Could you check a few things on this model? Use its own coordinates, in mm. A direction names the side the tool comes from. Coordinates: 2 decimals unless noted, no trailing zeros. Loops run counter-clockwise (first coordinate to the right, second up) from the corner with the lowest first, then second, coordinate; pieces in that order, holes last. Notation, with made-up numbers: (-24, 85.5) - (-14, 85.5) arc R26 ccw to (-14, 122.5) - close; hole circle Ø4 at (76, 75.25). An arc over 180 degrees is marked (long way). One line per question, with ' | ' between items. Start each with the question number.
1. We'd pull the mould along X, two halves only. Please class faces 3 (the flat face through (3.59, 0.746, 5.54)), 4 (the flat face through (0, -5, 0)): pulls with the +X half, pulls with the -X half, needs draft (parallel to the pull), parting line crosses it, or undercut.
2. I want a section at A-A, the plane x = 0. Write out the boundary of the cut face in (y, z).
3. I want a section at D-D, the plane x = -5.5. Write out the boundary of the cut face in (y, z).
4. I'm going to push flat-ended pins straight in: P1, Ø1.1, axis at x = -3, y = 4, coming from the +Z side; P2, Ø1.2, axis at y = 3, z = 6, coming from the +X side; P3, Ø3, axis at x = -4, z = 3, coming from the +Y side; P4, Ø1, axis at y = -1.5, z = 2, coming from the +X side. Where does each tip first touch, or does it pass through?
5. I want a section at B-B, the plane y = 0. Write out the boundary of the cut face in (x, z).
6. Please list where these lines run through material, in increasing order: L1, parallel to Y at x = 0, z = 0.7; L2, parallel to Y at x = 0, z = 2; L3, parallel to X at y = -0.5, z = 5.75. Write a range as [from, to].
7. I want a section at C-C, the plane y = -2.75. Write out the boundary of the cut face in (x, z).
8. Which directions (+Z, -Z, +X, -X, +Y, -Y) give clear straight access to the entire face, cutting with the end or side of a thin tool? Please do faces 1 (the flat face through (3.6, 0.223, 5.54)), 2 (the cylindrical face through (3.65, -2.8, 0.74)).
from build123d import *

# Parameters (mm, degrees)
SKETCH1_R           = 5.6
SKETCH1_R_2         = 1.5
BOSS_EXTRUDE1_DEPTH = 6.3
SKETCH2_R           = 1.7
CUT_EXTRUDE1_DEPTH  = 0.7
SKETCH3_R           = 5.1
SKETCH3_R_2         = 2.2
CUT_EXTRUDE2_DEPTH  = 1.5
BOSS_EXTRUDE2_DEPTH = 1.5
SKETCH5_R           = 4.6
SKETCH5_R_2         = 2.5
CUT_EXTRUDE3_DEPTH  = 1.5
BOSS_EXTRUDE4_START = -6.3
SKETCH6_R           = 7.35
SKETCH6_R_2         = 5.6
BOSS_EXTRUDE4_DEPTH = 6.3


with BuildPart() as part:
    # Sketch1 → Boss-Extrude1 (new body)
    with BuildSketch(Plane.XY):
        Circle(SKETCH1_R)
        Circle(SKETCH1_R_2, mode=Mode.SUBTRACT)
    extrude(amount=BOSS_EXTRUDE1_DEPTH)

    # Sketch2 → Cut-Extrude1 (cut)
    with BuildSketch(Plane.XY.offset(6.3)):
        Circle(SKETCH2_R)
    extrude(amount=-CUT_EXTRUDE1_DEPTH, mode=Mode.SUBTRACT)

    # Sketch3 → Cut-Extrude2 (cut)
    with BuildSketch(Plane.XY.offset(6.3)):
        Circle(SKETCH3_R)
        Circle(SKETCH3_R_2, mode=Mode.SUBTRACT)
    extrude(amount=-CUT_EXTRUDE2_DEPTH, mode=Mode.SUBTRACT)

    # Sketch4 → Boss-Extrude2 (add)
    with BuildSketch(Plane.XY.offset(4.8)):
        Polygon((-0.9, 2.00748599), (-0.9, 5.019960159), (-0.9, 5.084289528), (-0.4, 5.084289528), (-0.4, 2.163330765), (-0.4, 2.00748599), align=None)
        Polygon((0.4, 5.084289528), (0.4, 2.163330765), (0.4, 2.00748599), (0.9, 2.00748599), (0.9, 5.019960159), (0.9, 5.084289528), align=None)
        Polygon((1.631117337, 1.476298152), (4.496150526, 2.407203865), (4.557331391, 2.427082733), (4.711839888, 1.951554475), (1.933843023, 1.048928577), (1.785625834, 1.000769893), align=None)
        Polygon((2.03283943, 0.23992468), (2.187347927, -0.235603578), (5.052381116, 0.695302136), (5.113561981, 0.715181004), (4.959053484, 1.190709262), (2.181056619, 0.288083364), align=None)
        Polygon((1.908085954, -1.095083555), (3.678773844, -3.532226353), (3.716585698, -3.584269905), (3.3120772, -3.878162531), (1.595180717, -1.515057253), (1.503577457, -1.388976181), align=None)
        Polygon((0.856363861, -1.859204383), (0.451855364, -2.153097009), (2.222543254, -4.590239807), (2.260355108, -4.642283359), (2.664863605, -4.348390733), (0.947967122, -1.985285454), align=None)
        Polygon((-0.451855364, -2.153097009), (-2.222543254, -4.590239807), (-2.260355108, -4.642283359), (-2.664863605, -4.348390733), (-0.947967122, -1.985285454), (-0.856363861, -1.859204383), align=None)
        Polygon((-1.503577457, -1.388976181), (-1.908085954, -1.095083555), (-3.678773844, -3.532226353), (-3.716585698, -3.584269905), (-3.3120772, -3.878162531), (-1.595180717, -1.515057253), align=None)
        Polygon((-2.187347927, -0.235603578), (-5.052381116, 0.695302136), (-5.113561981, 0.715181004), (-4.959053484, 1.190709262), (-2.181056619, 0.288083364), (-2.03283943, 0.23992468), align=None)
        Polygon((-1.785625834, 1.000769893), (-1.631117337, 1.476298152), (-4.496150526, 2.407203865), (-4.557331391, 2.427082733), (-4.711839888, 1.951554475), (-1.933843023, 1.048928577), align=None)
    extrude(amount=BOSS_EXTRUDE2_DEPTH)

    # Sketch5 → Cut-Extrude3 (cut)
    with BuildSketch(Plane(origin=(0, 0, 0), x_dir=(-1, 0, 0), z_dir=(0, 0, -1))):
        Circle(SKETCH5_R)
        Circle(SKETCH5_R_2, mode=Mode.SUBTRACT)
    extrude(amount=-CUT_EXTRUDE3_DEPTH, mode=Mode.SUBTRACT)

    # Sketch6 → Boss-Extrude4 (add)
    with BuildSketch(Plane.XY.offset(6.3).offset(BOSS_EXTRUDE4_START)):
        Circle(SKETCH6_R)
        Circle(SKETCH6_R_2, mode=Mode.SUBTRACT)
    extrude(amount=BOSS_EXTRUDE4_DEPTH)


solid = part.part
Results are:
1) face 3: undercut | face 4: needs draft
2) outline: (-7.35, 0) - (-4.6, 0) - (-4.6, 1.5) - (-2.5, 1.5) - (-2.5, 0) - (-1.5, 0) - (-1.5, 5.6) - (-1.7, 5.6) - (-1.7, 6.3) - (-2.2, 6.3) - (-2.2, 4.8) - (-5.1, 4.8) - (-5.1, 6.3) - (-7.35, 6.3) - close; (1.5, 0) - (2.5, 0) - (2.5, 1.5) - (4.6, 1.5) - (4.6, 0) - (7.35, 0) - (7.35, 6.3) - (5.1, 6.3) - (5.1, 4.8) - (2.2, 4.8) - (2.2, 6.3) - (1.7, 6.3) - (1.7, 5.6) - (1.5, 5.6) - close
3) outline: (-4.88, 0) - (4.88, 0) - (4.88, 6.3) - (-4.88, 6.3) - close
4) P1: stops at z = 6.3 | P2: stops at x = 6.95 | P3: stops at y = 6.91 | P4: stops at x = 7.28
5) outline: (-7.35, 0) - (-4.6, 0) - (-4.6, 1.5) - (-2.5, 1.5) - (-2.5, 0) - (-1.5, 0) - (-1.5, 5.6) - (-1.7, 5.6) - (-1.7, 6.3) - (-2.91, 6.3) - (-2.91, 4.8) - (-5.1, 4.8) - (-5.1, 6.3) - (-7.35, 6.3) - close; (1.5, 0) - (2.5, 0) - (2.5, 1.5) - (4.6, 1.5) - (4.6, 0) - (7.35, 0) - (7.35, 6.3) - (5.1, 6.3) - (5.1, 4.8) - (2.91, 4.8) - (2.91, 6.3) - (1.7, 6.3) - (1.7, 5.6) - (1.5, 5.6) - close
6) L1: y = [-7.35, -4.6], [-2.5, -1.5], [1.5, 2.5], [4.6, 7.35] | L2: y = [-7.35, -1.5], [1.5, 7.35] | L3: x = [-7.33, -5.08], [-2.14, -1.62], [1.62, 2.14], [5.08, 7.33]
7) outline: (-6.82, 0) - (-3.69, 0) - (-3.69, 1.5) - (3.69, 1.5) - (3.69, 0) - (6.82, 0) - (6.82, 6.3) - (4.3, 6.3) - (4.3, 4.8) - (3.11, 4.8) - (3.11, 6.3) - (2.49, 6.3) - (2.49, 4.8) - (1.5, 4.8) - (1.5, 6.3) - (0.89, 6.3) - (0.89, 4.8) - (-0.89, 4.8) - (-0.89, 6.3) - (-1.5, 6.3) - (-1.5, 4.8) - (-2.49, 4.8) - (-2.49, 6.3) - (-3.11, 6.3) - (-3.11, 4.8) - (-4.3, 4.8) - (-4.3, 6.3) - (-6.82, 6.3) - close
8) face 1: +Z | face 2: -Z
